Solid Edge part; units mm, degrees
sketch "Sketch1" plane through (0, 0, 0) normal (0, 0, 1) x (1, 0, 0)
  line L0 (19, 25.318) -> (19, 15)
  line L1 (19, 15) -> (37.5, 15)
  arc A0 (37.5, 15) -> (38, 15.5) centre (37.5, 15.5) ccw
  line L2 (38, 15.5) -> (38, 19.557)
  line L3 (38, 19.557) -> (35.4486, 20.4958)
  line L4 (35.4486, 20.4958) -> (35.05, 19.4124)
  line L5 (35.05, 19.4124) -> (22.9816, 23.853)
  line L6 (22.9816, 23.853) -> (23.627, 25.607)
  line L7 (23.627, 25.607) -> (19.289, 25.607)
  arc A1 (19.289, 25.607) -> (19, 25.318) centre (19.289, 25.318) ccw
revolve "RevolvedProtrusion1" add sketch "Sketch1" angle 360 about axis through (50, 0, 0) along (-1, 0, 0)
Input: part model. Units: mm. Frame: model coordinates. A direction names the side the tool comes from. Coordinates: 2 decimals unless noted, no trailing zeros. Write each loop counter-clockwise with the first axis right and the second up, starting at its lowest first coordinate (ties: lowest second). Pieces come first, ordered by that corner, then holes. Notation, with made-up numbers: M -21.5,-18 L 23.5,-18 A14 ccw 23.5,8 Z; hole C -12.5,-29 d8. An arc over 180 degrees is marked long. Answer as a JSON object with one key per item and string values. Group by question number.
(1) Contact query for flat-ended pins moving along their axis: P1, Ø6, axis at x = 22, y = 13.5, coming from the +Z side; P2, Ø24, axis at y = 0, z = 0, coming from the -X side; P3, Ø10, axis at x = 35.5, y = 3, coming from the -Z side; P4, Ø2, axis at x = 34, y = 17, coming from the -Z side. Output: stop coordinate, or through.
(2) Mould query, pull axis Y, two halves, no side actions, for faces 1 (the face through (37.84, -4.25, 19.15)), 2 (the face through (19, 11, 11)), 3 (the face through (28.38, -14.985, 0.66)). Classes: pulls with the +Y half, pulls with the -Y half, needs draft (parallel to the pull), parting line crosses it, or undercut.
(3) Section D-D on x = 24.25. Output: boundary loops of the cut face in (y, z), plus the area to 3 significant figures.
(4) Section C-C on x = 29.25. Output: boundary loops of the cut face in (y, z), plus the area to 3 significant figures.
(5) Set-up query: faces 4 (the face through (34.3, 18.78, -5.91)), 5 (the face through (21.43, -5.55, 25)). Return all of +Z, -Z, +X, -X, +Y, -Y with unobstructed straight access to the full face (end or side cutting, diameter ignored); none if empty.
(6) Section A-A on y = 0. Output: boundary loops of the cut face in (x, z), plus the area to 3 significant figures.
(7) Ray query, line 1 along Z through (x, y) = (33.25, -10.5); line 2 along Z through (x, y) = (24.75, 0); line 3 along Y through (x, z) = (22.75, -4.5). Return the intervals inside material, ascending. Write a range as [from, to].
Result set:
{
 "1": {"P1": "stops at z = 23.36", "P2": "passes through", "P3": "stops at z = -20.96", "P4": "stops at z = -11.8"},
 "2": {"face 1": "parting line crosses it", "face 2": "needs draft", "face 3": "undercut"},
 "3": {"outline": "C 0,0 d46.77; hole C 0,0 d30", "area": "1,010 mm2"},
 "4": {"outline": "C 0,0 d43.09; hole C 0,0 d30", "area": "752 mm2"},
 "5": {"face 4": "none", "face 5": "+X, -X"},
 "6": {"outline": "M 19,-25.32 A0.29 ccw 19.29,-25.61 L 23.63,-25.61 L 22.98,-23.85 L 35.05,-19.41 L 35.45,-20.5 L 38,-19.56 L 38,-15.5 A0.5 ccw 37.5,-15 L 19,-15 Z; M 19,15 L 37.5,15 A0.5 ccw 38,15.5 L 38,19.56 L 35.45,20.5 L 35.05,19.41 L 22.98,23.85 L 23.63,25.61 L 19.29,25.61 A0.29 ccw 19,25.32 Z", "area": "275 mm2"},
 "7": {"line 1": "z = [-17.11, -10.71], [10.71, 17.11]", "line 2": "z = [-23.2, -15], [15, 23.2]", "line 3": "y = [-25.21, -14.31], [14.31, 25.21]"}
}
